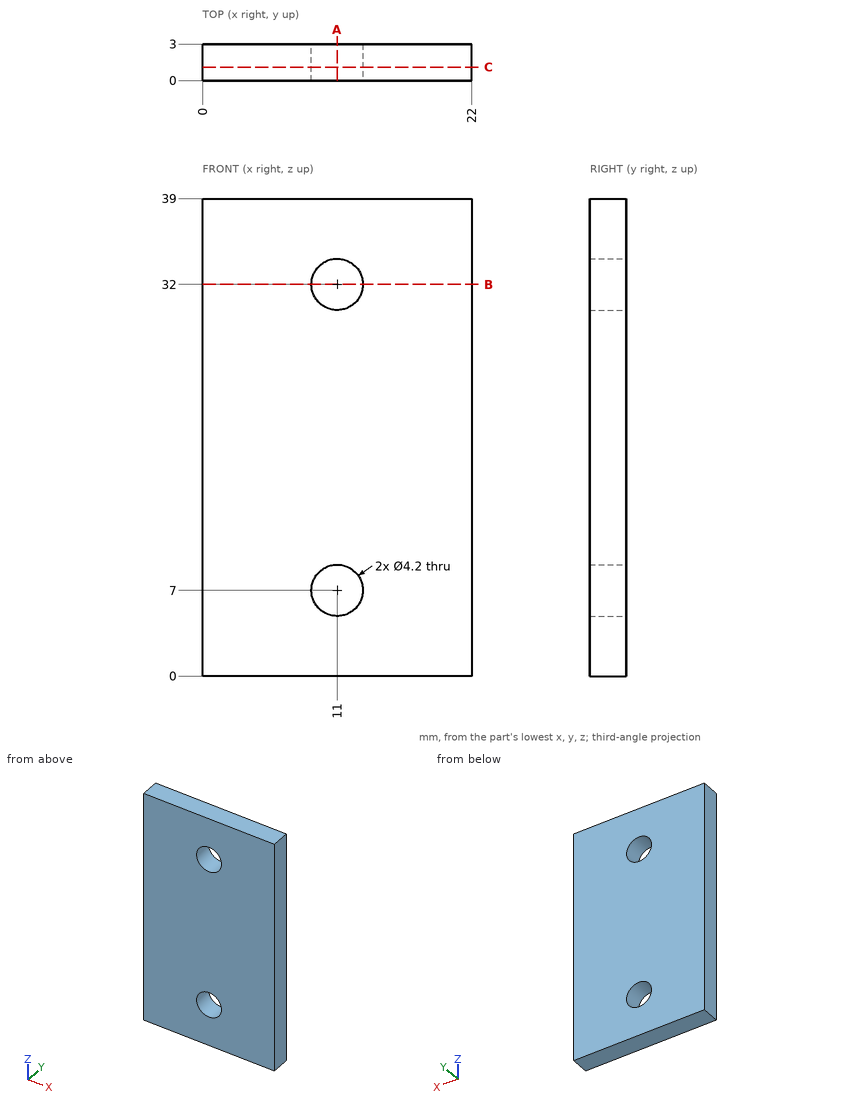
The figure shows three views and two pictorial views of one solid part (mm, origin at its lowest corner). Answer the questions. Coordinates: 2 decimals unless noted, no trailing zeros. Loops run counter-clockwise (first coordinate to the right, second up) from the corner with the lowest first, then second, coordinate; pieces in that order, holes last. Notation, with made-up numbers: (83.25, 48.25) -> (96.25, 48.25) arc R37 cw to (96.25, 84.25) -> close; hole circle Ø10 at (15.5, -13.75). An arc over 180 degrees is marked (long way). Return JSON: item names as keys, results as strings. Group by question number.
(1) A cutting plane is placed at B-B on z = 32. Write down the section's boundary in (x, y).
(2) A cutting plane is placed at C-C on y = 1.1. Write down the section's boundary in (x, z), and give its area (3 significant figures).
(3) A cutting plane is placed at A-A on x = 11. Write down the section's boundary in (y, z).
(4) Find the intervals of material crossed by probe 1 along Z at (x, y) = (11, 1.35); probe 2 along X at (y, z) = (1.25, 32); probe 3 along Z at (x, y) = (9.25, 0.2), in increasing order. Write a range as from..to.
The answers:
{
 "1": {"outline": "(0, 0) -> (8.9, 0) -> (8.9, 3) -> (0, 3) -> close; (13.1, 0) -> (22, 0) -> (22, 3) -> (13.1, 3) -> close"},
 "2": {"outline": "(0, 0) -> (22, 0) -> (22, 39) -> (0, 39) -> close; hole circle Ø4.2 at (11, 7); hole circle Ø4.2 at (11, 32)", "area": "830 mm^2"},
 "3": {"outline": "(0, 0) -> (3, 0) -> (3, 4.9) -> (0, 4.9) -> close; (0, 9.1) -> (3, 9.1) -> (3, 29.9) -> (0, 29.9) -> close; (0, 34.1) -> (3, 34.1) -> (3, 39) -> (0, 39) -> close"},
 "4": {"probe 1": "z = 0..4.9, 9.1..29.9, 34.1..39", "probe 2": "x = 0..8.9, 13.1..22", "probe 3": "z = 0..5.84, 8.16..30.84, 33.16..39"}
}
